Answer from the drawing. Dimensions are ordinates in mm from the lowest x, y and z of the part. Coordinates: 2 decimals unless noted, no trailing zeros. Write each loop counter-clockwise with the first axis right and the second up, starting at its lowest first coordinate (ties: lowest second). Pieces come first, ordered by that corner, then holes.
(1) Section C-C on x = 7 is taken. Write down the section's boundary in (y, z).
(2) Section A-A on z = 8 is taken. Write down the section's boundary in (x, y).
(3) Section D-D on x = 35 is taken. Write down the section's boundary in (y, z).
(4) Find the intervals of material crossed by probe 1 along X at (y, z) = (27, 8); probe 2 along X at (y, z) = (33, 7); probe 3 along Y at (x, z) = (43, 5.25), in increasing order.
(5) Section B-B on y = 20 is taken. Write down the section's boundary in (x, z), then the cut area to 3 significant figures.
(6) Given pin 1 (2.5 mm diameter, centred on x = 7, y = 20, fed in from -Z), flat-ended and moving along its own axis, determine where the tip first touches the part or whether it passes through.
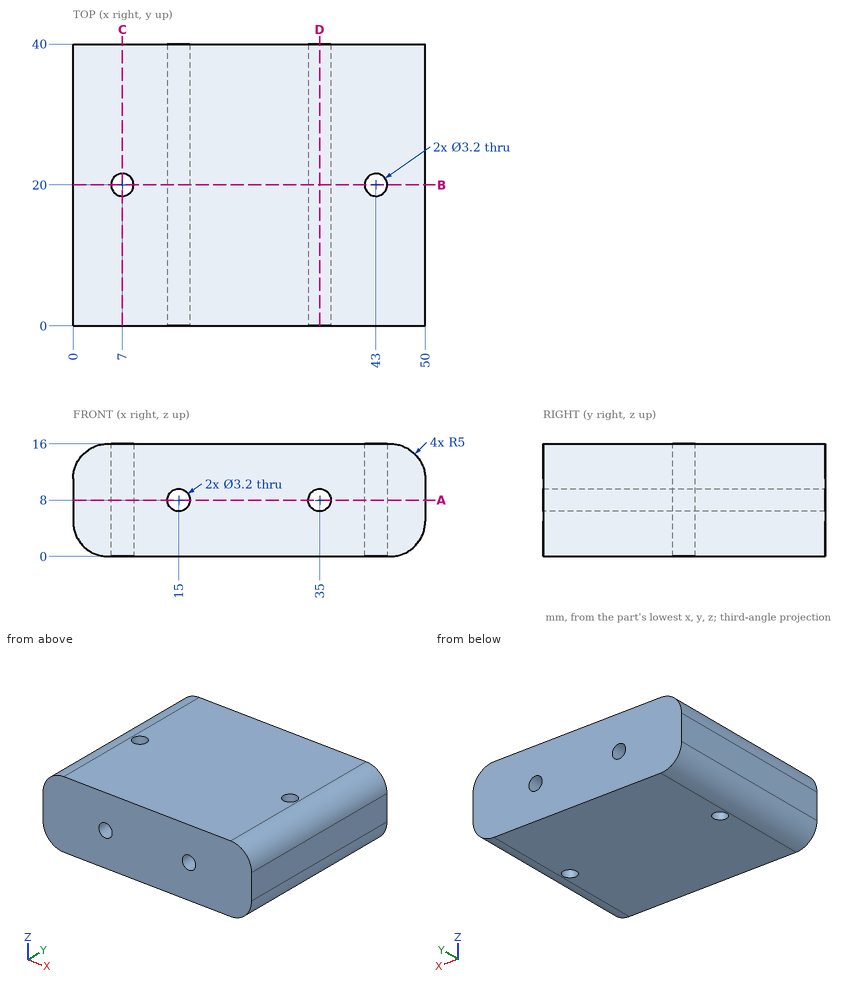
Response:
1. outline: (0, 0) - (18.4, 0) - (18.4, 16) - (0, 16) - close; (21.6, 0) - (40, 0) - (40, 16) - (21.6, 16) - close
2. outline: (0, 0) - (13.4, 0) - (13.4, 40) - (0, 40) - close; (16.6, 0) - (33.4, 0) - (33.4, 40) - (16.6, 40) - close; (36.6, 0) - (50, 0) - (50, 40) - (36.6, 40) - close; hole circle Ø3.2 at (7, 20); hole circle Ø3.2 at (43, 20)
3. outline: (0, 0) - (40, 0) - (40, 6.4) - (0, 6.4) - close; (0, 9.6) - (40, 9.6) - (40, 16) - (0, 16) - close
4. probe 1: x = 0 to 13.4, 16.6 to 33.4, 36.6 to 50
4. probe 2: x = 0 to 13.75, 16.25 to 33.75, 36.25 to 50
4. probe 3: y = 0 to 18.4, 21.6 to 40
5. outline: (0, 5) arc R5 ccw to (5, 0) - (5.4, 0) - (5.4, 16) - (5, 16) arc R5 ccw to (0, 11) - close; (8.6, 0) - (41.4, 0) - (41.4, 16) - (8.6, 16) - close; (44.6, 0) - (45, 0) arc R5 ccw to (50, 5) - (50, 11) arc R5 ccw to (45, 16) - (44.6, 16) - close; hole circle Ø3.2 at (15, 8); hole circle Ø3.2 at (35, 8)
5. area: 660 mm2
6. pin 1: passes through
